For this review, use the dimensioned drawing (mm, ordinates from the lowest corner) and the shaded views. A direction names the side the tool comes from. Give positions to 0.01 mm unless a question says otherwise; leave off trailing zeros. Order: outer loops, then holes, each group sorted by start corner. A loop starts at its lowest first (then second) coordinate and runs counter-clockwise, first axis right, second up.
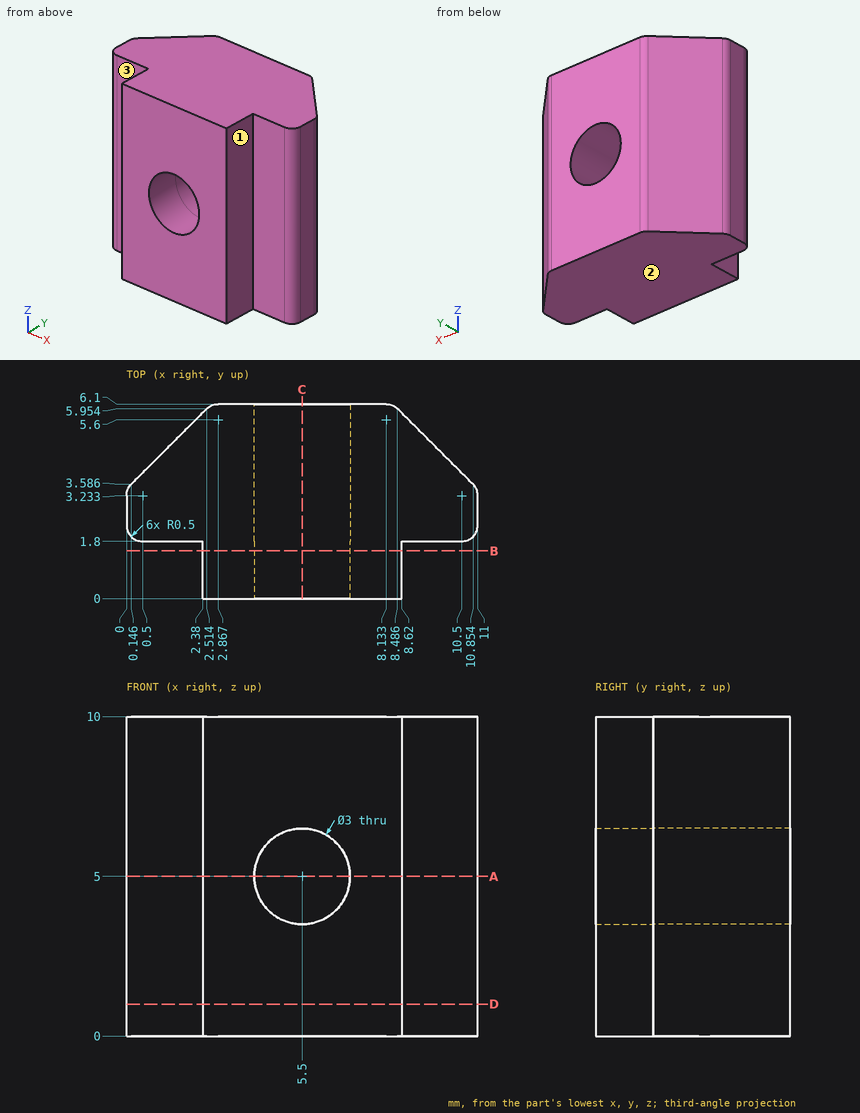
1. Machinability: for the marked faces 1, 2 and 3, which of the approach directions +Z, -Z, +X, -X, +Y, -Y give a long, thin tool a straight path to every point of the face, cutting with its end or side? Answer none if there is none.
Recorded:
face 1: +Z, -Z, +X, -Y
face 2: -Z, +X, -X, +Y, -Y
face 3: +Z, -Z, -X, -Y
2. Take a section at A-A (z = 5). State the section outline as (x, y) points.
Recorded:
outline: (0, 2.3) arc R0.5 ccw to (0.5, 1.8) - (2.38, 1.8) - (2.38, 0) - (4, 0) - (4, 6.1) - (2.87, 6.1) arc R0.5 ccw to (2.51, 5.95) - (0.15, 3.59) arc R0.5 ccw to (0, 3.23) - close; (7, 0) - (8.62, 0) - (8.62, 1.8) - (10.5, 1.8) arc R0.5 ccw to (11, 2.3) - (11, 3.23) arc R0.5 ccw to (10.85, 3.59) - (8.49, 5.95) arc R0.5 ccw to (8.13, 6.1) - (7, 6.1) - close
3. Take a section at C-C (x = 5.5). State the section outline as (y, z) points.
Recorded:
outline: (0, 0) - (6.1, 0) - (6.1, 3.5) - (0, 3.5) - close; (0, 6.5) - (6.1, 6.5) - (6.1, 10) - (0, 10) - close
4. Take a section at B-B (y = 1.5). State the section outline as (x, z) points.
Recorded:
outline: (2.38, 0) - (8.62, 0) - (8.62, 10) - (2.38, 10) - close; hole circle Ø3 at (5.5, 5)
5. For line 1 along Z through (x, y) = (5.5, 0.4); line 2 along X through (y, z) = (0.4, 5); line 3 along X through (y, z) = (3.4, 5), list the stretches that pass through material, from the lowest coordinate up.
Recorded:
line 1: z = 0 to 3.5, 6.5 to 10
line 2: x = 2.38 to 4, 7 to 8.62
line 3: x = 0.03 to 4, 7 to 10.97
6. For pin 1 (0.9 mm diameter, centred on y = 0.5, z = 3, fed in from -X); pin 2 (1.8 mm diameter, centred on x = 5.5, z = 5, fed in from +Y); pin 3 (0.6 mm diameter, centred on x = 1, z = 5, fed in from -Y); pin 4 (1 mm diameter, centred on y = 4, z = 4, fed in from +X), all flat-tipped, find the tip position at first contact; note any pin that passes through.
Recorded:
pin 1: stops at x = 2.38
pin 2: passes through
pin 3: stops at y = 1.8
pin 4: stops at x = 10.92
7. Take a section at D-D (z = 1). State the section outline as (x, y) points.
Recorded:
outline: (0, 2.3) arc R0.5 ccw to (0.5, 1.8) - (2.38, 1.8) - (2.38, 0) - (8.62, 0) - (8.62, 1.8) - (10.5, 1.8) arc R0.5 ccw to (11, 2.3) - (11, 3.23) arc R0.5 ccw to (10.85, 3.59) - (8.49, 5.95) arc R0.5 ccw to (8.13, 6.1) - (2.87, 6.1) arc R0.5 ccw to (2.51, 5.95) - (0.15, 3.59) arc R0.5 ccw to (0, 3.23) - close
